Could you check a few things on this model? Use its own coordinates, in mm. Coordinates: 2 decimals unless noted, no trailing zeros. Loops run counter-clockwise (first coordinate to the right, second up) from the corner with the lowest first, then second, coordinate; pieces in that order, holes last. Notation, with made-up numbers: (42, 8) -> (82, 8) arc R23 ccw to (82, 23) -> close; hole circle Ø1 at (32.5, -8). An arc over 180 degrees is marked (long way). One line per question, with ' | ' between items. Start each with the question number.
(1) If I drill on line 1 along X through (y, z) = (-41, 24); line 2 along Y through (x, z) = (92, 33); line 3 along Y through (x, z) = (69.5, 35.25), over which ranges is the centre line in solid material (lowest first)?
(2) Suppose I cut it at B-B (x = 49). Please give me the cut outline in (y, z).
(3) Suppose I cut it at A-A (y = -58). Please give me the cut outline in (x, z).
(4) I'm going to push flat-ended pins straight in: pin 1 Ø6 at (y, z) = (-47, 15.5) entering from +X; pin 2 Ø1.5 at (x, z) = (72.5, 23) entering from +Y; pin 3 Ø10 at (y, z) = (-72.5, 27) entering from +X. Where does each tip first touch, or does it pass through?
(5) Suppose I cut it at D-D (x = 87). Please give me the cut outline in (y, z).
(6) Suppose I cut it at C-C (z = 20.25). Please give me the cut outline in (x, y).
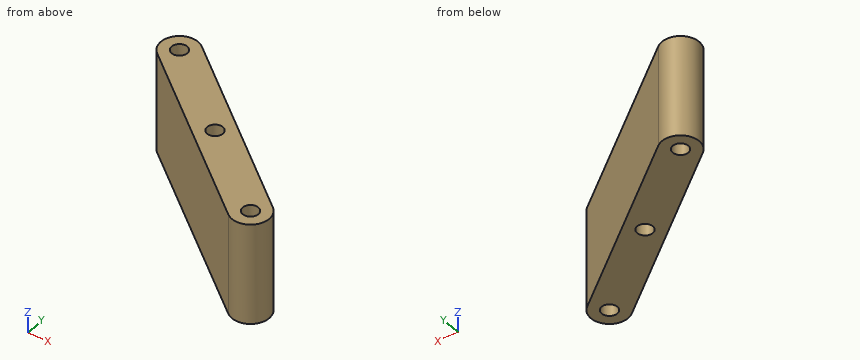
```python
from build123d import *

# Parameters (mm, degrees)
SKETCH1_R           = 2.1
BOSS_EXTRUDE1_DEPTH = 27


with BuildPart() as part:
    # Sketch1 → Boss-Extrude1 (new body)
    with BuildSketch(Plane.XY.offset(10)):
        with BuildLine():
            Line((44.663839647, -44.004447821), (90.626506234, -82.571704402))
            ThreePointArc((90.626506234, -82.571704402), (97.670666498, -81.955420235), (97.054382331, -74.911259971))
            Line((97.054382331, -74.911259971), (51.091715743, -36.34400339))
            ThreePointArc((51.091715743, -36.34400339), (44.047555479, -36.960287557), (44.663839647, -44.004447821))
        make_face()
        with Locations((47.877777695, -40.174225605)):
            Circle(SKETCH1_R, mode=Mode.SUBTRACT)
        with Locations((70.859110989, -59.457853896)):
            Circle(SKETCH1_R, mode=Mode.SUBTRACT)
        with Locations((93.840444282, -78.741482187)):
            Circle(SKETCH1_R, mode=Mode.SUBTRACT)
    extrude(amount=BOSS_EXTRUDE1_DEPTH)


solid = part.part
```
Checks:
1) line 1: x = 42.95 to 45.95, 49.81 to 56.64 | line 2: y = -83.39 to -79.75, -77.73 to -70.67 | line 3: y = -64.84 to -61.06, -57.86 to -51.79
2) outline: (-47.64, 10) -> (-41.95, 10) -> (-41.95, 37) -> (-47.64, 37) -> close; (-38.4, 10) -> (-35.3, 10) -> (-35.3, 37) -> (-38.4, 37) -> close
3) outline: (61.34, 10) -> (69.35, 10) -> (69.35, 37) -> (61.34, 37) -> close; (72.37, 10) -> (76.9, 10) -> (76.9, 37) -> (72.37, 37) -> close
4) pin 1: stops at x = 67.37 | pin 2: stops at y = -53.68 | pin 3: stops at x = 98.68
5) outline: (-79.53, 10) -> (-66.47, 10) -> (-66.47, 37) -> (-79.53, 37) -> close
6) outline: (44.66, -44) -> (90.63, -82.57) arc R5 ccw to (97.05, -74.91) -> (51.09, -36.34) arc R5 ccw to start; hole circle Ø4.2 at (47.88, -40.17); hole circle Ø4.2 at (70.86, -59.46); hole circle Ø4.2 at (93.84, -78.74)
